Part model, mm, in its own coordinate system. Round coordinates to 2 decimals unless told otherwise and drop trailing zeros. Order: outer loops, then holes, each group sorted by start corner. A loop starts at its lowest first (then second) coordinate and runs counter-clockwise, first axis right, second up. Notation, with made-up numbers: (-8, -4) -> (29, -4) arc R22 ccw to (29, 19) -> close; hole circle Ø3 at (-17, 19). An arc over 180 degrees is marked (long way). Return JSON: item names as keys, results as strings. Group by question number.
from build123d import *

# Parameters (mm, degrees)
SKETCH1_W           = 64.012274628
SKETCH1_H           = 75.085000506
BOSS_EXTRUDE1_DEPTH = 5
SKETCH7_R           = 1.4732
CUT_EXTRUDE1_DEPTH  = 10


with BuildPart() as part:
    # Sketch1 → Boss-Extrude1 (new body)
    # profile 1 of 2: a face of its own
    with BuildSketch(Plane.XY):
        with Locations((61.398411242, 7.077500224)):
            Rectangle(SKETCH1_W, SKETCH1_H)
        with BuildLine():
            ThreePointArc((83.484398078, 2.429730903), (59.871437613, -17.479677368), (44.238109553, 9.157805497))
            ThreePointArc((44.238109553, 9.157805497), (59.81501285, 35.930775127), (83.520814038, 15.994205484))
            ThreePointArc((83.520814038, 15.994205484), (83.22114917, 12.52456978), (82.331029644, 9.157693158))
            ThreePointArc((82.331029644, 9.157693158), (83.193968093, 5.842784333), (83.484398078, 2.429730903))
        make_face(mode=Mode.SUBTRACT)
    # profile 2 of 2: a face of its own
    with BuildSketch(Plane.XY):
        with Locations((-2.613863386, 7.077500224)):
            Rectangle(SKETCH1_W, SKETCH1_H)
        with BuildLine():
            ThreePointArc((15.69984642, 2.429730903), (-7.913055331, -17.479687433), (-23.546481788, 9.157693158))
            ThreePointArc((-23.546481788, 9.157693158), (-7.969677608, 35.930764895), (15.736182375, 15.994205484))
            ThreePointArc((15.736182375, 15.994205484), (15.436527739, 12.524628574), (14.546438303, 9.157805497))
            ThreePointArc((14.546438303, 9.157805497), (15.409406369, 5.842843047), (15.69984642, 2.429730903))
        make_face(mode=Mode.SUBTRACT)
    extrude(amount=BOSS_EXTRUDE1_DEPTH)

    # Sketch7 → Cut-Extrude1 (cut)
    with BuildSketch(Plane.XY.offset(5)):
        with Locations((-23.500584488, 33.499560055)):
            Circle(SKETCH7_R)
        with Locations((14.49941543, 33.50027263)):
            Circle(SKETCH7_R)
        with Locations((-23.49959354, -19.345440441)):
            Circle(SKETCH7_R)
        with Locations((14.500406379, -19.344727866)):
            Circle(SKETCH7_R)
        with Locations((44.284829686, -19.345328379)):
            Circle(SKETCH7_R)
        with Locations((44.284150424, 33.499672122)):
            Circle(SKETCH7_R)
        with Locations((82.284150347, 33.500160568)):
            Circle(SKETCH7_R)
        with Locations((82.284829608, -19.344839933)):
            Circle(SKETCH7_R)
    extrude(amount=-CUT_EXTRUDE1_DEPTH, mode=Mode.SUBTRACT)


solid = part.part
(1) Saw through at C-C, the plane z = 2.4. State how many separate pieces and enclosed holes the cut face has, and give its area (3 significant figures).
(2) Pin check, flat tip, straight feed: P1, Ø4.5, axis at x = 44.28, y = 33.5, coming from the +Z side. Stop position of the tip, or through.
(3) Probe L1, parallel to X at y = 16, z = 1.05; L2, parallel to X at y = 26.5, z = 4.4; L3, parallel to Y at x = 59, z = 1.65 (1 decimal). List the from-to ranges inside material, lowest first. Write a range as [from, to].
(4) Saw through at A-A, the plane y = 12. List the corners of the cut face in (x, z), and give its area (3 significant figures).
(5) Saw through at D-D, the plane y = 28.5. List the corners of the cut face in (x, z), and give its area (3 significant figures).
(6) Mould opens along X. For faces 1 (the cylindrical face through (83.646, -19.909, 2.535)), 2 (the flat face through (93.405, 7, 2)), 3 (the flat face through (28, 44.62, 2)) say: pulls with the +X half, pulls with the -X half, needs draft (parallel to the pull), parting line crosses it, or undercut.
(7) Saw through at B-B, the plane x = 69.5. List the corners of the cut face in (y, z) (3 decimals).
Results are:
{
 "1": {"separate pieces": "1", "enclosed holes": "10", "area": "5,910 mm^2"},
 "2": {"P1": "stops at z = 5"},
 "3": {"L1": "x = [-34.62, -24.74], [15.74, 43.05], [83.52, 93.4]", "L2": "x = [-34.62, -21.8], [12.8, 45.99], [80.58, 93.4]", "L3": "y = [-30.5, -17.3], [35.8, 44.6]"},
 "4": {"outline": "(-34.62, 0) -> (-24.34, 0) -> (-24.34, 5) -> (-34.62, 5) -> close; (15.34, 0) -> (43.45, 0) -> (43.45, 5) -> (15.34, 5) -> close; (83.12, 0) -> (93.4, 0) -> (93.4, 5) -> (83.12, 5) -> close", "area": "243 mm^2"},
 "5": {"outline": "(-34.62, 0) -> (-20.41, 0) -> (-20.41, 5) -> (-34.62, 5) -> close; (11.41, 0) -> (47.38, 0) -> (47.38, 5) -> (11.41, 5) -> close; (79.19, 0) -> (93.4, 0) -> (93.4, 5) -> (79.19, 5) -> close", "area": "322 mm^2"},
 "6": {"face 1": "undercut", "face 2": "pulls with the +X half", "face 3": "needs draft"},
 "7": {"outline": "(-30.465, 0) -> (-16.79, 0) -> (-16.79, 5) -> (-30.465, 5) -> close; (35.252, 0) -> (44.62, 0) -> (44.62, 5) -> (35.252, 5) -> close"}
}
